Here's the drawing with two shaded views (mm, measured from the low corner). I have some questions. Coordinates: 2 decimals unless noted, no trailing zeros. Write each loop counter-clockwise with the first axis right and the second up, starting at its lowest first coordinate (ties: lowest second). Pieces come first, ordered by that corner, then holes. Notation, with made-up numbers: (-10, -27) - (6, -27) arc R33 cw to (6, 9) - close; hole circle Ø5 at (81.25, 81.5). An arc over 180 degrees is marked (long way). Answer in a Markdown table with one row per item. Add a question column.
Item 1: Imagine slicing it at B-B (x = 20). Please give me the cut outline in (y, z).
Item 2: Imagine slicing it at A-A (y = 25). Please give me the cut outline in (x, z).
Item 3: I'm going to push a flat-ended pin straight in: pin 1 (5 mm diameter, centred on x = 30, y = 15, fed in from -Z). Where does the tip first touch, or does it pass through?
Item 4: If I drill on probe 1 along Y at (x, z) = (40, 4.75); probe 2 along Y at (x, z) = (50, 8); probe 3 along X at (y, z) = (37.5, 2.25), over which ranges is the centre line in solid material (lowest first)? Write a range as from..to.
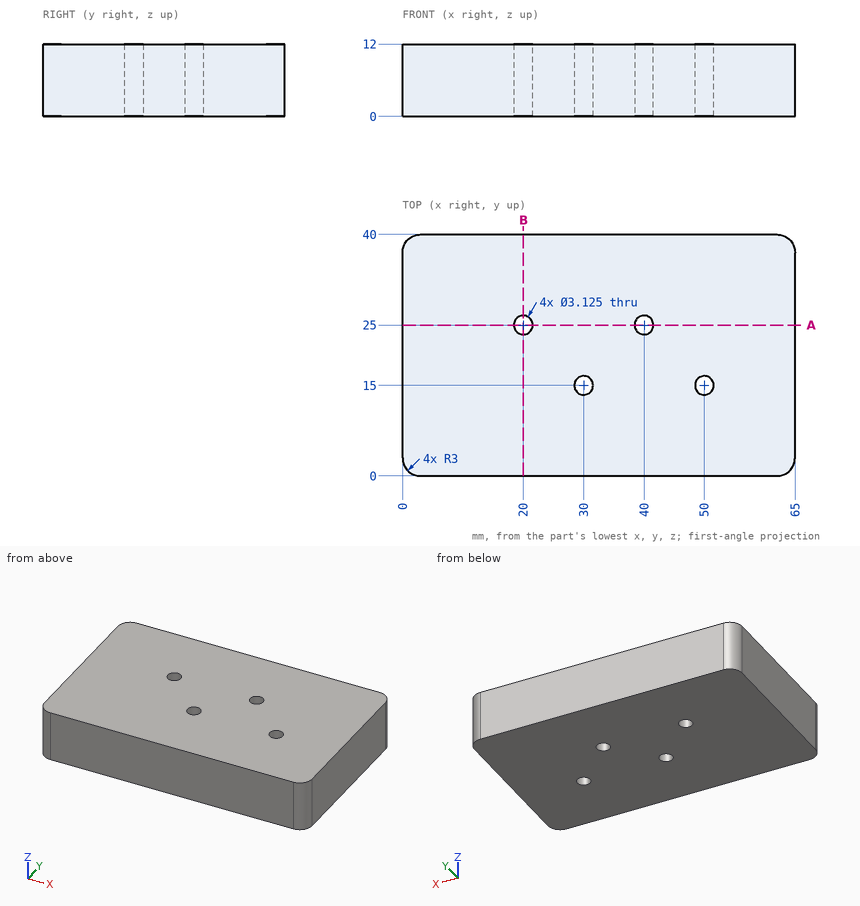
Here are the results:
| question | item | result |
|---|---|---|
| 1 | outline | (0, 0) - (23.44, 0) - (23.44, 12) - (0, 12) - close; (26.56, 0) - (40, 0) - (40, 12) - (26.56, 12) - close |
| 2 | outline | (0, 0) - (18.44, 0) - (18.44, 12) - (0, 12) - close; (21.56, 0) - (38.44, 0) - (38.44, 12) - (21.56, 12) - close; (41.56, 0) - (65, 0) - (65, 12) - (41.56, 12) - close |
| 3 | pin 1 | stops at z = 0 |
| 4 | probe 1 | y = 0..23.44, 26.56..40 |
| 4 | probe 2 | y = 0..13.44, 16.56..40 |
| 4 | probe 3 | x = 0.04..64.96 |
